The listing builds one solid part. Answer for the finished solid, in the listing's coordinates (mm). Face numbers are marked on the shaded views. A direction names the side the tool comes from. Give positions to 0.01 mm unless a question says otherwise; leave off trailing zeros. Order: outer loops, then holes, each group sorted by start corner. A loop starts at its lowest first (then second) coordinate and runs counter-clockwise, first axis right, second up.
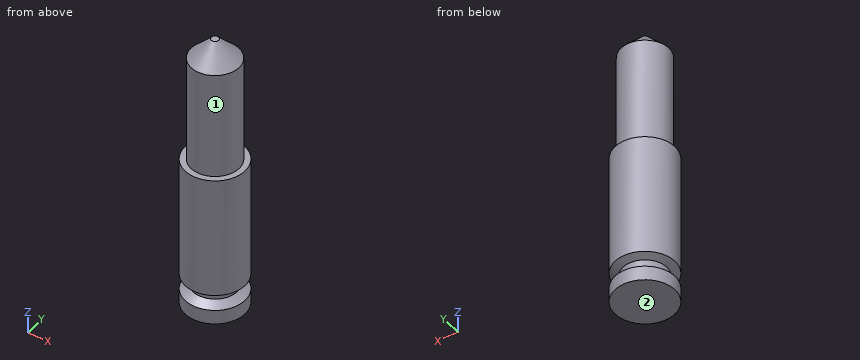
Autodesk Inventor part; units mm, degrees
ref_plane "YZ Plane" through (0, 0, 0) normal (1, 0, 0) x (0, 1, 0)
ref_plane "XZ Plane" through (0, 0, 0) normal (0, 1, 0) x (-1, 0, 0)
ref_plane "XY Plane" through (0, 0, 0) normal (0, 0, 1) x (1, 0, 0)
sketch "Sketch1" plane through (0, 0, 0) normal (0, 1, 0) x (-1, 0, 0)
  line L0 (0, 0) -> (-7.9629, 0)
  line L1 (-7.9629, 0) -> (-7.9629, 3.81)
  line L2 (-7.9629, 3.81) -> (-5.842, 5.334)
  line L3 (-5.842, 5.334) -> (-5.842, 7.239)
  line L4 (-5.842, 7.239) -> (-7.9629, 8.001)
  line L5 (-7.9629, 8.001) -> (-7.9629, 40.259)
  line L6 (-7.9629, 40.259) -> (-6.3754, 40.259)
  line L7 (-6.3754, 40.259) -> (-6.3754, 68.6656)
  line L8 (-6.3754, 68.6656) -> (-1, 74.041)
  line L9 (-1, 74.041) -> (0, 74.041)
  line L10 (0, 74.041) -> (0, 0)
  dimension "d1" = 3.81
  dimension "d3" = 74.041
  dimension "d4" = 32.258
  dimension "d5" = 0.762
  dimension "d6" = 1.524
  dimension "d7" = 4.191
  dimension "d8" = 5.842
  dimension "d9" = 7.9629
  dimension "d10" = 6.3754
  dimension "d11" = 45
  dimension "d12" = 1
revolve "Revolution1" add sketch "Sketch1" angle 360 about axis through (0, 0, 74.041) along (0, 0, -1)
properties part number "ubis"
1) A tool of negligible diameter and unlimited length cuts with its end or side. For the marked faces 1 and 2, from which of +Z, -Z, +X, -X, +Y, -Y can it reach the whole face along a straight path? Write none if from no direction.
Geometry says:
face 1: +Z
face 2: -Z, +X, -X, +Y, -Y
2) Find section A-A (x = 0). Write down the section's boundary in (y, z), then the cut area to 3 significant figures.
Geometry says:
outline: (-7.96, 0) - (7.96, 0) - (7.96, 3.81) - (5.84, 5.33) - (5.84, 7.24) - (7.96, 8) - (7.96, 40.26) - (6.38, 40.26) - (6.38, 68.67) - (1, 74.04) - (-1, 74.04) - (-6.38, 68.67) - (-6.38, 40.26) - (-7.96, 40.26) - (-7.96, 8) - (-5.84, 7.24) - (-5.84, 5.33) - (-7.96, 3.81) - close
area: 1,030 mm2
3) Given P1, Ø4, axis at y = -3.5, z = 60.5, coming from the -X side; P2, Ø5, axis at y = 6, z = 50.5, coming from the +X side; P3, Ø4, axis at y = 5, z = 34.5, coming from the +X side, each flat-ended and moving along its own axis, determine where each tip first touches the part or whether it passes through.
Geometry says:
P1: stops at x = -6.2
P2: stops at x = 5.33
P3: stops at x = 7.38
4) Straight lines are drawn through the part: probe 1 along Y at (x, z) = (0, 53.5); probe 2 along Z at (x, y) = (2.75, -5.5); probe 3 along Z at (x, y) = (5.5, -2.25). For each, find the intervals that lie inside material, in ascending order.
Geometry says:
probe 1: y = -6.38 to 6.38
probe 2: z = 0 to 5.11, 7.35 to 68.89
probe 3: z = 0 to 5.26, 7.28 to 69.1
5) Find section C-C (z = 38). Write down the section's boundary in (x, y), then the cut area to 3 significant figures.
Geometry says:
outline: circle Ø15.93 at (0, 0)
area: 199 mm2
